Verification items for the finished model (mm, model axes). Round coordinates to 2 decimals unless told otherwise and drop trailing zeros. Order: outer loops, then holes, each group sorted by start corner. A loop starts at its lowest first (then second) coordinate and runs counter-clockwise, first axis right, second up. Notation, with made-up numbers: (55.25, -28.75) -> (101.25, -28.75) arc R30 ccw to (101.25, -5.75) -> close; hole circle Ø1 at (44, 40). An arc over 180 degrees is marked (long way). Put each result on its own line as item: value.
Solid Edge part; units mm, degrees
sketch "Sketch1" plane through (0, 0, 0) normal (0, 0, 1) x (1, 0, 0)
  line L0 (13.8251, 10.4054) -> (65.3251, 10.4054)
  line L1 (59.5751, 21.5054) -> (65.3251, 10.4054)
  line L2 (39.5751, 21.5054) -> (59.5751, 21.5054)
  line L3 (39.5751, 21.5054) -> (19.5751, 21.5054)
  line L4 (19.5751, 21.5054) -> (13.8251, 10.4054)
extrude "Protrusion1" add sketch "Sketch1" along normal blind 4
hole "Furo_1" at (31.3751, 14.5054, 4) direction (0, 0, -1) diameter 3 end up to next
hole "Hole1" at (47.1751, 14.5054, 4) direction (0, 0, -1) diameter 3 end up to next
fillet "Redondo_1" radius 5 2 edges at (59.5751, 21.5054, 2) (19.5751, 21.5054, 2)
Item 1: Depth check by flat-ended pin: pin 1 Ø2.5 at (x, y) = (31.38, 14.51) entering from +Z; pin 2 Ø2 at (y, z) = (19, 1) entering from +X. Enter the tip coordinate at first touch or a pass-through.
Geometry check:
pin 1: through
pin 2: x = 61.39
Item 2: Sectioned sample at D-D, the plane x = 46.5. Record the boundary of the cut face in (y, z).
Geometry check:
outline: (10.41, 0) -> (13.17, 0) -> (13.17, 4) -> (10.41, 4) -> close; (15.84, 0) -> (21.51, 0) -> (21.51, 4) -> (15.84, 4) -> close
Item 3: Release check for a two-part mould opening along X. For faces 1 (the face through (40, 21.505, 2)), 2 (the face through (59.16, 20.76, 2.03)), 3 (the face through (48.662, 14.701, 2.028)) record: pulls with the +X half, pulls with the -X half, needs draft (parallel to the pull), parting line crosses it, or undercut.
Geometry check:
face 1: needs draft
face 2: pulls with the +X half
face 3: undercut
Item 4: Sectioned sample at B-B, the plane y = 14.5. Record the boundary of the cut face in (x, z), then the cut area to 3 significant figures.
Geometry check:
outline: (15.95, 0) -> (29.88, 0) -> (29.88, 4) -> (15.95, 4) -> close; (32.88, 0) -> (45.68, 0) -> (45.68, 4) -> (32.88, 4) -> close; (48.68, 0) -> (63.2, 0) -> (63.2, 4) -> (48.68, 4) -> close
area: 165 mm2
Item 5: Sectioned sample at C-C, the plane z = 2.2. Record the boundary of the cut face in (x, y).
Geometry check:
outline: (13.83, 10.41) -> (65.33, 10.41) -> (60.97, 18.81) arc R5 ccw to (56.53, 21.51) -> (22.62, 21.51) arc R5 ccw to (18.18, 18.81) -> close; hole circle Ø3 at (31.38, 14.51); hole circle Ø3 at (47.18, 14.51)
Item 6: Material ranges on line 1 along X through (y, z) = (14.5, 1.85); line 2 along X through (y, z) = (13.75, 3.75); line 3 along X through (y, z) = (12, 1.7), recorded low to high.
Geometry check:
line 1: 15.95 to 29.88, 32.88 to 45.68, 48.68 to 63.2
line 2: 15.56 to 30.08, 32.67 to 45.88, 48.47 to 63.59
line 3: 14.65 to 64.5
Item 7: Sectioned sample at A-A, the plane x = 32. Record the boundary of the cut face in (y, z).
Geometry check:
outline: (10.41, 0) -> (13.14, 0) -> (13.14, 4) -> (10.41, 4) -> close; (15.87, 0) -> (21.51, 0) -> (21.51, 4) -> (15.87, 4) -> close
